Could you check a few things on this model? Use its own coordinates, in mm. A direction names the side the tool comes from. Give positions to 0.01 mm unless a question says otherwise; leave off trailing zeros. Write each loop counter-clockwise with the first axis right and the second up, starting at its lowest first coordinate (ties: lowest second). Pieces come first, ordered by that corner, then holes. Notation, with made-up numbers: (85.25, 39) - (124.25, 39) arc R12 cw to (124.25, 58) - close; hole circle Ø11 at (-14, -2). An arc over 180 degrees is marked (long way). Answer in a Markdown table with one row per item.
from build123d import *

# Parameters (mm, degrees)
F0_W     = 25
F0_H     = 16
F0_W_2   = 21.8
F0_H_2   = 13.2
F1_DEPTH = 0.3
F2_DEPTH = 0.6
F3_R     = 1
F4_R     = 0.5


with BuildPart() as f1:
    # F0 (on Top) → F1 (new body)
    with BuildSketch(Plane.XY):
        Rectangle(F0_W, F0_H)
        Rectangle(F0_W_2, F0_H_2, mode=Mode.SUBTRACT)
        Rectangle(F0_W_2, F0_H_2)
    extrude(amount=F1_DEPTH)

    # F0 (on Top) → F2 (join)
    with BuildSketch(Plane.XY):
        Rectangle(F0_W_2, F0_H_2)
    extrude(amount=F2_DEPTH)

    # F3
    f3_edges = [f1.edges().sort_by_distance(p)[0] for p in [
        (-12.5, 8, 0.15),
        (-12.5, -8, 0.15),
        (12.5, -8, 0.15),
        (12.5, 8, 0.15),
    ]]
    fillet(f3_edges, radius=F3_R)

    # F4
    f4_edges = [f1.edges().sort_by_distance(p)[0] for p in [
        (-10.9, -6.6, 0.45),
        (10.9, -6.6, 0.45),
        (-10.9, 6.6, 0.45),
        (10.9, 6.6, 0.45),
    ]]
    fillet(f4_edges, radius=F4_R)


solid = f1.part
1) On a 3-axis mill with a long thin cutter (end or side, diameter ignored), from which of +Z, -Z, +X, -X, +Y, -Y can I reach the whole of each face in a straight line? I mean faces 1 (the face through (0, -7, 0.3)), 2 (the face through (0, 0, 0)). Say none if no direction works.
Check values:
| item | result |
|---|---|
| face 1 | +Z |
| face 2 | -Z, +X, -X, +Y, -Y |
2) Will this pin go through, and if not, where does the flat tip stop? P1, Ø2, axis at x = 3, y = -0.5, coming from the -Z side.
Check values:
| item | result |
|---|---|
| P1 | stops at z = 0 |
3) If I drill on line 1 (X direction, y = -2, z = 0.5); line 2 (Y direction, x = -8.25, z = 0.35); line 3 (Z direction, x = -11, y = -3.75), over which ranges is the centre line in solid material (lowest first)?
Check values:
| item | result |
|---|---|
| line 1 | x = -10.9 to 10.9 |
| line 2 | y = -6.6 to 6.6 |
| line 3 | z = 0 to 0.3 |
4) Imagine slicing it at B-B (y = -4.75). List the corners of the cut face in (x, z) for me.
Check values:
| item | result |
|---|---|
| outline | (-12.5, 0) - (12.5, 0) - (12.5, 0.3) - (10.9, 0.3) - (10.9, 0.6) - (-10.9, 0.6) - (-10.9, 0.3) - (-12.5, 0.3) - close |
5) Imagine slicing it at A-A (z = 0.45). List the corners of the cut face in (x, y) for me, then the cut area to 3 significant figures.
Check values:
| item | result |
|---|---|
| outline | (-10.9, -6.1) arc R0.5 ccw to (-10.4, -6.6) - (10.4, -6.6) arc R0.5 ccw to (10.9, -6.1) - (10.9, 6.1) arc R0.5 ccw to (10.4, 6.6) - (-10.4, 6.6) arc R0.5 ccw to (-10.9, 6.1) - close |
| area | 288 mm2 |
